```python
from build123d import *

# Parameters (mm, degrees)
F0_W      = 700
F0_H      = 700
F0_W_2    = 600
F0_H_2    = 600
F1_DEPTH  = 50
F2_W      = 50
F2_H      = 50
F3_DEPTH  = 700
F4_W      = 700
F4_H      = 700
F4_W_2    = 600
F4_H_2    = 600
F5_DEPTH  = 50
F6_W      = 100
F6_H      = 50
F6_W_2    = 50
F6_H_2    = 100
F7_DEPTH  = 50
F8_W      = 50
F8_H      = 50
F9_DEPTH  = 700
F10_W     = 700
F10_H     = 700
F10_W_2   = 600
F10_H_2   = 600
F11_DEPTH = 50
F12_W     = 50
F12_H     = 50
F13_DEPTH = 500
F14_W     = 100
F14_H     = 50
F14_W_2   = 50
F14_H_2   = 100
F15_DEPTH = 50
F16_W     = 600
F16_H     = 50
F17_DEPTH = 50
F18_W     = 100
F18_H     = 50
F18_W_2   = 50
F18_H_2   = 100
F19_DEPTH = 50


with BuildPart() as f1:
    # F0 (on Top) → F1 (new body)
    with BuildSketch(Plane.XY):
        Rectangle(F0_W, F0_H)
        Rectangle(F0_W_2, F0_H_2, mode=Mode.SUBTRACT)
    extrude(amount=-F1_DEPTH)

    # F2 (on face) → F3 (join)
    with BuildSketch(Plane(origin=(0, 0, -50), x_dir=(1, 0, 0), z_dir=(0, 0, -1))):
        with Locations((-325, 325)):
            Rectangle(F2_W, F2_H)
        with Locations((325, 325)):
            Rectangle(F2_W, F2_H)
        with Locations((325, -325)):
            Rectangle(F2_W, F2_H)
        with Locations((-325, -325)):
            Rectangle(F2_W, F2_H)
    extrude(amount=F3_DEPTH)

    # F4 (on face) → F5 (join)
    with BuildSketch(Plane(origin=(0, 0, -750), x_dir=(1, 0, 0), z_dir=(0, 0, -1))):
        Rectangle(F4_W, F4_H)
        Rectangle(F4_W_2, F4_H_2, mode=Mode.SUBTRACT)
    extrude(amount=F5_DEPTH)

    # F6 (on face) → F7 (join)
    with BuildSketch(Plane.XY):
        with Locations((-250, 0)):
            Rectangle(F6_W, F6_H)
        with Locations((0, -250)):
            Rectangle(F6_W_2, F6_H_2)
        with Locations((250, 0)):
            Rectangle(F6_W, F6_H)
        with Locations((0, 250)):
            Rectangle(F6_W_2, F6_H_2)
    extrude(amount=-F7_DEPTH)

    # F8 (on face) → F9 (join)
    with BuildSketch(Plane(origin=(0, 0, -800), x_dir=(1, 0, 0), z_dir=(0, 0, -1))):
        with Locations((-325, 325)):
            Rectangle(F8_W, F8_H)
        with Locations((325, 325)):
            Rectangle(F8_W, F8_H)
        with Locations((-325, -325)):
            Rectangle(F8_W, F8_H)
        with Locations((325, -325)):
            Rectangle(F8_W, F8_H)
    extrude(amount=F9_DEPTH)

    # F10 (on face) → F11 (join)
    with BuildSketch(Plane(origin=(0, 0, -1500), x_dir=(1, 0, 0), z_dir=(0, 0, -1))):
        Rectangle(F10_W, F10_H)
        Rectangle(F10_W_2, F10_H_2, mode=Mode.SUBTRACT)
    extrude(amount=F11_DEPTH)

    # F12 (on face) → F13 (join)
    with BuildSketch(Plane(origin=(0, 0, -1550), x_dir=(1, 0, 0), z_dir=(0, 0, -1))):
        with Locations((-325, 325)):
            Rectangle(F12_W, F12_H)
        with Locations((325, 325)):
            Rectangle(F12_W, F12_H)
        with Locations((-325, -325)):
            Rectangle(F12_W, F12_H)
        with Locations((325, -325)):
            Rectangle(F12_W, F12_H)
    extrude(amount=F13_DEPTH)

    # F14 (on face) → F15 (join)
    with BuildSketch(Plane.XY.offset(-750)):
        with Locations((-250, 0)):
            Rectangle(F14_W, F14_H)
        with Locations((0, -250)):
            Rectangle(F14_W_2, F14_H_2)
        with Locations((250, 0)):
            Rectangle(F14_W, F14_H)
        with Locations((0, 250)):
            Rectangle(F14_W_2, F14_H_2)
    extrude(amount=-F15_DEPTH)

    # F16 (on face) → F17 (cut, through all)
    with BuildSketch(Plane.XY.offset(-1500)):
        with Locations((0, -325)):
            Rectangle(F16_W, F16_H)
    extrude(amount=-F17_DEPTH, mode=Mode.SUBTRACT)

    # F18 (on face) → F19 (join)
    with BuildSketch(Plane.XY.offset(-1500)):
        with Locations((-250, 0)):
            Rectangle(F18_W, F18_H)
        with Locations((250, 0)):
            Rectangle(F18_W, F18_H)
        with Locations((0, 250)):
            Rectangle(F18_W_2, F18_H_2)
    extrude(amount=-F19_DEPTH)


solid = f1.part
```
For this review, take the finished solid that the model builds, in its own axes (mm). A direction names the side the tool comes from. Round coordinates to 2 decimals unless told otherwise and drop trailing zeros. Loops run counter-clockwise (first coordinate to the right, second up) from the corner with the lowest first, then second, coordinate; pieces in that order, holes last.
(1) Wall thickness on line 1 along Z through (x, y) = (-245, 0); line 2 along Y through (x, z) = (-315.5, -418); line 3 along Z through (x, y) = (-14, -283): over which ranges is each line inside the solid? List them lowest first.
Returned:
line 1: z = -1550 to -1500, -800 to -750, -50 to 0
line 2: y = -350 to -300, 300 to 350
line 3: z = -800 to -750, -50 to 0
(2) Tool access review of faces 1 (the flat face through (-164, 300, -25)), 2 (the flat face through (249, -25, -1525)), 3 (the flat face through (-300, 325, -395)): name each direction out of +Z, -Z, +X, -X, +Y, -Y from which nothing blocks a thin tool from reaching the whole face with its end or side.
Returned:
face 1: +Z, -Z
face 2: +Z, -Z, -Y
face 3: +Y, -Y
(3) We need section D-D (y = -250.5). State how many separate pieces and enclosed holes the cut face has, plus the area to 3 significant figures.
Returned:
separate pieces: 8
enclosed holes: 0
area: 20,000 mm2
(4) Mouldability with a two-part tool opening along Z and no side actions: class faces 4 (the flat face through (-164, 300, -1525)), 5 (the flat face through (-325, 325, -2050)), 6 (the flat face through (-4, 307, -1500)) as released by +Z, released by -Z, zero draft, split by the parting line, or undercut.
Returned:
face 4: zero draft
face 5: released by -Z
face 6: undercut
(5) We need section A-A (y = 2.5). Give the boundary of the cut face in (x, z), plus the area to 3 significant figures.
Returned:
outline: (-350, -1550) - (-200, -1550) - (-200, -1500) - (-350, -1500) - close; (-350, -800) - (-200, -800) - (-200, -750) - (-350, -750) - close; (-350, -50) - (-200, -50) - (-200, 0) - (-350, 0) - close; (200, -1550) - (350, -1550) - (350, -1500) - (200, -1500) - close; (200, -800) - (350, -800) - (350, -750) - (200, -750) - close; (200, -50) - (350, -50) - (350, 0) - (200, 0) - close
area: 45,000 mm2
(6) We need section B-B (x = 124). Give the boundary of the cut face in (y, z).
Returned:
outline: (-350, -800) - (-300, -800) - (-300, -750) - (-350, -750) - close; (-350, -50) - (-300, -50) - (-300, 0) - (-350, 0) - close; (300, -1550) - (350, -1550) - (350, -1500) - (300, -1500) - close; (300, -800) - (350, -800) - (350, -750) - (300, -750) - close; (300, -50) - (350, -50) - (350, 0) - (300, 0) - close
(7) We need section C-C (z = -582). Give the boundary of the cut face in (x, y), plus the area to 3 significant figures.
Returned:
outline: (-350, -350) - (-300, -350) - (-300, -300) - (-350, -300) - close; (-350, 300) - (-300, 300) - (-300, 350) - (-350, 350) - close; (300, -350) - (350, -350) - (350, -300) - (300, -300) - close; (300, 300) - (350, 300) - (350, 350) - (300, 350) - close
area: 10,000 mm2
